Could you check a few things on this model? Use its own coordinates, in mm. A direction names the side the tool comes from. Give positions to 0.01 mm unless a question says otherwise; leave off trailing zeros. Write each loop counter-clockwise with the first axis right and the second up, starting at its lowest first coordinate (ties: lowest second). Pieces come first, ordered by that corner, then holes. Notation, with made-up numbers: (18, 45.5) - (25, 45.5) arc R8 cw to (25, 55.5) - close; hole circle Ø1 at (66.25, 10.5). An arc over 180 degrees is marked (long way). Write item = value, one per line.
from build123d import *

# Parameters (mm, degrees)
SZKIC1_W                    = 36
SZKIC1_H                    = 16
DODANIE_WYCI_GNI_CIE1_DEPTH = 6
WYTNIJ_WYCI_GNI_CIE1_DEPTH  = 6
SZKIC3_R                    = 1.55
WYTNIJ_WYCI_GNI_CIE2_DEPTH  = 74.51650454


with BuildPart() as part:
    # Szkic1 → Dodanie-wyciągnięcie1 (new body)
    with BuildSketch(Plane.XY):
        with Locations((53.502982034, -8)):
            Rectangle(SZKIC1_W, SZKIC1_H)
    extrude(amount=-DODANIE_WYCI_GNI_CIE1_DEPTH)

    # Szkic2 → Wytnij-wyciągnięcie1 (cut)
    with BuildSketch(Plane.XY):
        with BuildLine():
            Line((55.002982034, -4.065016704), (55.002982034, -2.5))
            Line((55.002982034, -2.5), (52.002982034, -2.5))
            Line((52.002982034, -2.5), (52.002982034, -4.065016704))
            ThreePointArc((52.002982034, -4.065016704), (46.727022487, -9.497551457), (49.612982034, -16.498938498))
            Line((49.612982034, -16.498938498), (49.612982034, -16))
            Line((49.612982034, -16), (57.392982034, -16))
            Line((57.392982034, -16), (57.392982034, -16.498938498))
            ThreePointArc((57.392982034, -16.498938498), (60.278941582, -9.497551457), (55.002982034, -4.065016704))
        make_face()
    extrude(amount=-WYTNIJ_WYCI_GNI_CIE1_DEPTH, mode=Mode.SUBTRACT)

    # Szkic3 → Wytnij-wyciągnięcie2 (cut, through all)
    with BuildSketch(Plane(origin=(0, 0, -6), x_dir=(-1, 0, 0), z_dir=(0, 0, -1))):
        with Locations((-44.502982035, -12)):
            Circle(SZKIC3_R)
        with Locations((-44.502982035, -4)):
            Circle(SZKIC3_R)
        with Locations((-62.502982035, -4)):
            Circle(SZKIC3_R)
        with Locations((-62.502982035, -12)):
            Circle(SZKIC3_R)
    extrude(amount=-WYTNIJ_WYCI_GNI_CIE2_DEPTH, mode=Mode.SUBTRACT)


solid = part.part
1. For pin 1 (6 mm diameter, centred on x = 44, y = -9, fed in from +Z); pin 2 (3.5 mm diameter, centred on x = 54, z = -2.5, fed in from -Y); pin 3 (2 mm diameter, centred on x = 57, z = -4, fed in from -Y), each with a flat end and sliding along its axis, tell me the tip position at first contact or that it passes through.
Filled sheet:
pin_1 = 0
pin_2 = -4.28
pin_3 = -5.57
2. I need wall thicknesses on line 1 (Y direction, x = 62.5, z = -3.25); line 2 (X direction, y = -12.5, z = -2.1); line 3 (Y direction, x = 63.5, z = -0.7). Which ranges of each line are inside material? Lowest first, please.
Filled sheet:
line_1 = -16 to -13.55, -10.45 to -5.55, -2.45 to 0
line_2 = 35.5 to 43.04, 45.97 to 46.82, 60.19 to 61.04, 63.97 to 71.5
line_3 = -16 to -13.19, -10.81 to -5.19, -2.81 to 0
3. If we section it at C-C, the plane y = -3.25: Please give me the cut outline in (x, z).
Filled sheet:
outline = (35.5, -6) - (43.15, -6) - (43.15, 0) - (35.5, 0) - close; (45.86, -6) - (52, -6) - (52, 0) - (45.86, 0) - close; (55, -6) - (61.15, -6) - (61.15, 0) - (55, 0) - close; (63.86, -6) - (71.5, -6) - (71.5, 0) - (63.86, 0) - close
4. Which directions (+Z, -Z, +X, -X, +Y, -Y) give clear straight access to the entire face, cutting with the end or side of a thin tool? Please do faces 4 (the face through (60.216, -9.203, -2.958)), 5 (the face through (52.003, -3, -3)), 6 (the face through (57, -4, -6)).
Filled sheet:
face_4 = +Z, -Z
face_5 = +Z, -Z, -Y
face_6 = -Z, +X, -X, +Y, -Y
5. Thinking about a two-plate mould opening in Y: for faces 1 (the face through (61.025, -11.534, -3.042)), 2 (the face through (42, -16, -3)), 3 (the face through (57, -4, 0)), which applies, pulls with the +Y half, pulls with the -Y half, needs draft (parallel to the pull), parting line crosses it, or undercut?
Filled sheet:
face_1 = undercut
face_2 = pulls with the -Y half
face_3 = needs draft
6. If we section it at D-D, the plane y = -9.75: Please give me the cut outline in (x, z), and give its area (3 significant figures).
Filled sheet:
outline = (35.5, -6) - (46.68, -6) - (46.68, 0) - (35.5, 0) - close; (60.32, -6) - (71.5, -6) - (71.5, 0) - (60.32, 0) - close
area = 134 mm2
7. If we section it at A-A, the plane z = -2.2: Please give me the cut outline in (x, y).
Filled sheet:
outline = (35.5, -16) - (48.97, -16) arc R6.9 cw to (52, -4.07) - (52, -2.5) - (55, -2.5) - (55, -4.07) arc R6.9 cw to (58.04, -16) - (71.5, -16) - (71.5, 0) - (35.5, 0) - close; hole circle Ø3.1 at (44.5, -12); hole circle Ø3.1 at (44.5, -4); hole circle Ø3.1 at (62.5, -12); hole circle Ø3.1 at (62.5, -4)
8. If we section it at B-B, the plane x = 58.5: Please give me the cut outline in (y, z).
Filled sheet:
outline = (-16, -6) - (-15.56, -6) - (-15.56, 0) - (-16, 0) - close; (-6.04, -6) - (0, -6) - (0, 0) - (-6.04, 0) - close
